For this review, take the finished solid that the model builds, in its own axes (mm). A direction names the side the tool comes from. Coordinates: 2 decimals unless noted, no trailing zeros. Write each loop counter-clockwise with the first axis right and the second up, starting at its lowest first coordinate (ties: lowest second). Pieces come first, ordered by that corner, then holes. Notation, with made-up numbers: (18, 55.5) -> (34, 55.5) arc R11 cw to (34, 68.5) -> close; hole circle Ø2 at (39.25, -26.75). An arc over 180 degrees is marked (long way). Put each result on its own line as item: value. Start each with the question number.
Item 1: Consider section A-A on x = 5.25. Give the boundary of the cut face in (y, z).
Item 2: Insertion check: P1, Ø1.6, axis at x = 7, y = 8, coming from the +Z side; P2, Ø3, axis at y = -5.66, z = 5.66, coming from the +X side. Each pin has a flat end and moves straight along its axis. Give the tip position at first contact, or say it passes through.
Item 3: Consider section B-B on y = 0. Give the boundary of the cut face in (x, z).
Item 4: Consider section C-C on z = 0. Give the boundary of the cut face in (x, y).
Item 5: Consider section D-D on x = 7.75. Give the boundary of the cut face in (y, z), and give its area (3 significant figures).
Item 6: For faces 1 (the flat face through (7, 0, 16.15)), 2 (the cylindrical face through (1.48, 2.23, 0.29)), list the 3-axis set-ups (+Z, -Z, +X, -X, +Y, -Y) from which the entire face can be reached by the end or side of a thin tool; tool diameter is ignored.
Item 7: To check wall thickness, follow L1, parallel to Y at x = 7, z = -18.35; L2, parallel to Y at x = 2.5, z = -5.5; L3, parallel to Z at x = 2.75, y = 6.5. State the ranges of each line that lie inside material, in increasing order.
Item 8: The part is to be moulded in two halves that separate along Z. For faces 3 (the flat face through (5, 0, 19.15)), 4 (the cylindrical face through (1.48, -6.73, 5.9)), 5 (the flat face through (5, 0, -19.15)), say which applies: +Z half, -Z half, draft (parallel to the pull), parting line (faces both ways), or undercut.
```python
from build123d import *

# Parameters (mm, degrees)
SKETCH1_W           = 32.3
SKETCH1_H           = 22.5
SKETCH1_R           = 1.1
SKETCH1_R_2         = 2.25
BOSS_EXTRUDE1_DEPTH = 3
SKETCH1_5_W         = 3
SKETCH1_5_H         = 22.5
BOSS_EXTRUDE5_DEPTH = 10.3
CUT_EXTRUDE1_REACH  = 43.226
SKETCH2_R           = 1.35


with BuildPart() as part:
    # Sketch1 → Boss-Extrude1 (new body)
    with BuildSketch(Plane(origin=(0, 0, 0), x_dir=(0, 0, -1), z_dir=(1, 0, 0))):
        Rectangle(SKETCH1_W, SKETCH1_H)
        with Locations((-5.656854249, -5.656854249)):
            Circle(SKETCH1_R, mode=Mode.SUBTRACT)
        with Locations((5.656854249, -5.656854249)):
            Circle(SKETCH1_R, mode=Mode.SUBTRACT)
        Circle(SKETCH1_R_2, mode=Mode.SUBTRACT)
        with Locations((-5.656854249, 5.656854249)):
            Circle(SKETCH1_R, mode=Mode.SUBTRACT)
        with Locations((5.656854249, 5.656854249)):
            Circle(SKETCH1_R, mode=Mode.SUBTRACT)
    extrude(amount=BOSS_EXTRUDE1_DEPTH)

    # Sketch1<5> → Boss-Extrude5 (add)
    with BuildSketch(Plane(origin=(0, 0, 0), x_dir=(0, 0, -1), z_dir=(1, 0, 0))):
        with Locations((17.65, 0)):
            Rectangle(SKETCH1_5_W, SKETCH1_5_H)
        with Locations((-17.65, 0)):
            Rectangle(SKETCH1_5_W, SKETCH1_5_H)
    extrude(amount=BOSS_EXTRUDE5_DEPTH)

    # Cut-Extrude1: up to this face of the body (flat: up to its plane)
    cut_extrude1_end = Plane(part.part.faces().sort_by_distance((5.15, 0, -19.15))[0])
    # Sketch2 → Cut-Extrude1 (cut, up to the picked face)
    with BuildSketch(Plane.XY.offset(19.15), mode=Mode.PRIVATE) as cut_extrude1_sk1:
        with Locations((7, 8)):
            Circle(SKETCH2_R)
    cut_extrude1_tool1 = split(extrude(cut_extrude1_sk1.sketch, amount=-CUT_EXTRUDE1_REACH, mode=Mode.PRIVATE), bisect_by=cut_extrude1_end, keep=Keep.BOTH, mode=Mode.PRIVATE)
    cut_extrude1 = cut_extrude1_tool1.solids().sort_by(Axis((7, 8, 19.15), (0, 0, -1)))[0]
    add(cut_extrude1, mode=Mode.SUBTRACT)

    # Mirror1: Cut-Extrude1 across plane
    add(cut_extrude1.mirror(Plane.ZX), mode=Mode.SUBTRACT)


solid = part.part
```
Return value:
1. outline: (-11.25, -19.15) -> (11.25, -19.15) -> (11.25, -16.15) -> (-11.25, -16.15) -> close; (-11.25, 16.15) -> (11.25, 16.15) -> (11.25, 19.15) -> (-11.25, 19.15) -> close
2. P1: through
2. P2: x = 3
3. outline: (0, -19.15) -> (10.3, -19.15) -> (10.3, -16.15) -> (3, -16.15) -> (3, -2.25) -> (0, -2.25) -> close; (0, 2.25) -> (3, 2.25) -> (3, 16.15) -> (10.3, 16.15) -> (10.3, 19.15) -> (0, 19.15) -> close
4. outline: (0, -11.25) -> (3, -11.25) -> (3, -2.25) -> (0, -2.25) -> close; (0, 2.25) -> (3, 2.25) -> (3, 11.25) -> (0, 11.25) -> close
5. outline: (-11.25, -19.15) -> (-9.12, -19.15) -> (-9.12, -16.15) -> (-11.25, -16.15) -> close; (-11.25, 16.15) -> (-9.12, 16.15) -> (-9.12, 19.15) -> (-11.25, 19.15) -> close; (-6.88, -19.15) -> (6.88, -19.15) -> (6.88, -16.15) -> (-6.88, -16.15) -> close; (-6.88, 16.15) -> (6.88, 16.15) -> (6.88, 19.15) -> (-6.88, 19.15) -> close; (9.12, -19.15) -> (11.25, -19.15) -> (11.25, -16.15) -> (9.12, -16.15) -> close; (9.12, 16.15) -> (11.25, 16.15) -> (11.25, 19.15) -> (9.12, 19.15) -> close
5. area: 108 mm^2
6. face 1: +X, +Y, -Y
6. face 2: +X, -X
7. L1: -11.25 to -9.35, -6.65 to 6.65, 9.35 to 11.25
7. L2: -11.25 to -6.75, -4.57 to 4.57, 6.75 to 11.25
7. L3: -19.15 to -6.36, -4.95 to 4.95, 6.36 to 19.15
8. face 3: +Z half
8. face 4: undercut
8. face 5: -Z half
